Verification items for the finished model (mm, model axes). A direction names the side the tool comes from. Coordinates: 2 decimals unless noted, no trailing zeros. Loops run counter-clockwise (first coordinate to the right, second up) from the corner with the lowest first, then second, coordinate; pieces in that order, holes last.
Q1. Mould release check, pull along X, two halves, no side actions. Record for faces 3 (the face through (152.4, -2, 6)), 4 (the face through (-2, -152.4, 6)), 5 (the face through (-152.4, -2, 6)), 6 (the face through (-36.534, -28.013, 6.261)): +X half, -X half, draft (parallel to the pull), parting line (faces both ways), or undercut.
Q2. Sectioned sample at A-A (x = 0). Enter the section's corners in (y, z), then the cut area to 3 significant figures.
Q3. Access from +Z, -Z, +X, -X, +Y, -Y to the whole of each face (thin tool, end or side, straight path). Record for faces 1 (the face through (-2, 152.4, 6)), 2 (the face through (72, -72, 9.525)).
Q4. Material ranges on probe 1 along Y at (x, z) = (0, 4.5); probe 2 along X at (y, z) = (25, 4.5); probe 3 along Y at (x, z) = (35, 5.5), recorded low to high.
Q5. Sectioned sample at C-C (z = 3.5). Enter the section's corners in (x, y) (1 decimal).
```python
from build123d import *

# Parameters (mm, degrees)
SKETCH1_W           = 304.8
SKETCH1_H           = 304.8
SKETCH1_R           = 46.0375
BOSS_EXTRUDE1_DEPTH = 12.7
SKETCH2_R           = 7.9375
CUT_EXTRUDE1_DEPTH  = 9.525


with BuildPart() as part:
    # Sketch1 → Boss-Extrude1 (new body)
    with BuildSketch(Plane.XY):
        Rectangle(SKETCH1_W, SKETCH1_H)
        Circle(SKETCH1_R, mode=Mode.SUBTRACT)
    extrude(amount=BOSS_EXTRUDE1_DEPTH)

    # Sketch2 → Cut-Extrude1 (cut)
    with BuildSketch(Plane.XY):
        with Locations(Location((-71.842048969, 71.842048969, 0), (0, 0, 180))):
            Circle(SKETCH2_R)
        with Locations(Location((71.842048969, -71.842048969, 0), (0, 0, 180))):
            Circle(SKETCH2_R)
    extrude(amount=CUT_EXTRUDE1_DEPTH, mode=Mode.SUBTRACT)


solid = part.part
```
Geometry check:
1. face 3: +X half
1. face 4: draft
1. face 5: -X half
1. face 6: undercut
2. outline: (-152.4, 0) - (-46.04, 0) - (-46.04, 12.7) - (-152.4, 12.7) - close; (46.04, 0) - (152.4, 0) - (152.4, 12.7) - (46.04, 12.7) - close
2. area: 2,700 mm2
3. face 1: +Z, -Z, +X, -X, +Y
3. face 2: -Z
4. probe 1: y = -152.4 to -46.04, 46.04 to 152.4
4. probe 2: x = -152.4 to -38.66, 38.66 to 152.4
4. probe 3: y = -152.4 to -29.91, 29.91 to 152.4
5. outline: (-152.4, -152.4) - (152.4, -152.4) - (152.4, 152.4) - (-152.4, 152.4) - close; hole circle Ø15.9 at (-71.8, 71.8); hole circle Ø92.1 at (0, 0); hole circle Ø15.9 at (71.8, -71.8)
